Input: part model. Units: mm. Frame: model coordinates. Face numbers are marked on the shaded views. A direction names the side the tool comes from. Coordinates: 2 decimals unless noted, no trailing zeros. Loops run counter-clockwise (first coordinate to the right, second up) from the corner with the lowest first, then second, coordinate; pieces in that order, holes last. Notation, with made-up numbers: (16.5, 70) - (36.5, 70) arc R8 cw to (36.5, 81) - close; hole circle Ø6 at (37.5, 76.5). An arc over 180 degrees is marked (long way). Use a Markdown table: item, result. Add a question column.
1. Ray query, L1, parallel to Z at x = 41, y = -11 (3 decimals); L2, parallel to Z at x = -18, y = -16 (3 decimals); L3, parallel to X at y = -9, z = 42 (3 decimals). Return the intervals inside material, ascending. Write a range as [from, to].
2. Section query B-B on x = 0. Return the cut outline in (y, z) (1 decimal).
3. Section query C-C on z = 33.5. Return the cut outline in (x, y) (3 decimals), then the cut area to 3 significant figures.
4. Access query for the marked faces 1 and 2. Directions: +Z, -Z, +X, -X, +Y, -Y. A direction counts if a zero-diameter tool reaches every point of the face in a straight line with its end or side. Return the directions, or none.
5. Contact query for flat-ended pins moving along their axis: P1, Ø0.8, axis at x = 37, z = -71.5, coming from the -Y side; P2, Ø3, axis at x = 35, z = 72, coming from the -Y side; P3, Ø11, axis at y = -12.5, z = 66, coming from the -X side. Output: stop coordinate, or through.
6. Section query A-A on y = -7. Return the cut outline in (x, z) (3 decimals).
7. Draft query along X for the marked faces 3, 4 and 5. Return one class per face: released by +X, released by -X, zero draft, split by the parting line, or undercut.
```python
from build123d import *

# Parameters (mm, degrees)
SKETCH1_W               = 107.95
SKETCH1_H               = 146.05
BOSS_EXTRUDE1_DEPTH     = 2.54
SKETCH13_W              = 25.4
SKETCH13_H              = 25.4
BOSS_EXTRUDE4_DEPTH     = 19.431
SKETCH2_R               = 3.302
CUT_EXTRUDE1_DEPTH      = 93.862882849
FILLET1_R               = 12.7
CUT_EXTRUDE13_DEPTH     = 5.08
SKETCH15_R              = 6.35
BOSS_EXTRUDE5_DEPTH     = 11.811
SKETCH23_R              = 2.25
CUT_EXTRUDE14_DEPTH     = 92.934228941
SKETCH24_R              = 4
CUT_EXTRUDE15_DEPTH     = 3.81
MIRROR2_COPY_1_SKETCH_R = 2.25
MIRROR2_COPY_1_DEPTH    = 92.934228941
MIRROR2_COPY_2_SKETCH_R = 4
MIRROR2_COPY_2_DEPTH    = 3.81
FILLET3_R               = 12.7
FILLET4_R               = 1.016
SKETCH27_W              = 71.841582164
SKETCH27_H              = 2.54
SKETCH27_W_2            = 2.54
SKETCH27_H_2            = 108.293882364
BOSS_EXTRUDE6_DEPTH     = 33.782
CUT_EXTRUDE16_DEPTH     = 41.656
CUT_EXTRUDE17_DEPTH     = 136.296492227
CUT_EXTRUDE18_DEPTH     = 160.8849299
CUT_EXTRUDE19_REACH     = 161.885
SKETCH31_W              = 22.225
SKETCH31_H              = 12.7
FILLET5_R               = 2.54


with BuildPart() as part:
    # Sketch1 → Boss-Extrude1 (new body)
    with BuildSketch(Plane(origin=(0, 0, 0), x_dir=(1, 0, 0), z_dir=(0, 1, 0))):
        Rectangle(SKETCH1_W, SKETCH1_H)
    extrude(amount=-BOSS_EXTRUDE1_DEPTH)

    # Sketch13 → Boss-Extrude4 (add)
    with BuildSketch(Plane(origin=(0, 0, 0), x_dir=(1, 0, 0), z_dir=(0, 1, 0))):
        with Locations((41.275, -60.325)):
            Rectangle(SKETCH13_W, SKETCH13_H)
        with Locations((-41.275, -60.325)):
            Rectangle(SKETCH13_W, SKETCH13_H)
        with Locations((-41.275, 60.325)):
            Rectangle(SKETCH13_W, SKETCH13_H)
        with Locations((41.275, 60.325)):
            Rectangle(SKETCH13_W, SKETCH13_H)
    extrude(amount=-BOSS_EXTRUDE4_DEPTH)

    # Sketch2 → Cut-Extrude1 (cut, through all)
    with BuildSketch(Plane(origin=(0, 0, 0), x_dir=(1, 0, 0), z_dir=(0, 1, 0))):
        with Locations(Location((-41.275, 60.325, 0), (0, 0, 270))):
            Circle(SKETCH2_R)
        with Locations(Location((41.275, 60.325, 0), (0, 0, 90))):
            Circle(SKETCH2_R)
        with Locations(Location((41.275, -60.325, 0), (0, 0, 270))):
            Circle(SKETCH2_R)
        with Locations(Location((-41.275, -60.325, 0), (0, 0, 90))):
            Circle(SKETCH2_R)
    extrude(amount=-CUT_EXTRUDE1_DEPTH, mode=Mode.SUBTRACT)

    # Fillet1
    fillet1_edges = [part.edges().sort_by_distance(p)[0] for p in [
        (53.975, -9.7155, 73.025),
        (-53.975, -9.7155, 73.025),
        (-53.975, -9.7155, -73.025),
        (53.975, -9.7155, -73.025),
    ]]
    fillet(fillet1_edges, radius=FILLET1_R)

    # Sketch14 → Cut-Extrude13 (cut)
    with BuildSketch(Plane.XZ.offset(19.431)):
        Polygon((20.692003582, -28.674172721), (6.35, -45.983487389), (139.336989519, -156.172707277), (153.678993101, -138.863392609), align=None)
        Polygon((-20.692003582, -28.674172721), (-6.35, -45.983487389), (-139.336989519, -156.172707277), (-153.678993101, -138.863392609), align=None)
        Polygon((-153.678993101, 138.863392609), (-20.692003582, 28.674172721), (-6.35, 45.983487389), (-139.336989519, 156.172707277), align=None)
        Polygon((20.692003582, 28.674172721), (6.35, 45.983487389), (139.336989519, 156.172707277), (153.678993101, 138.863392609), align=None)
    extrude(amount=-CUT_EXTRUDE13_DEPTH, mode=Mode.SUBTRACT)

    # Sketch15 → Boss-Extrude5 (add)
    with BuildSketch(Plane(origin=(0, 0, 0), x_dir=(1, 0, 0), z_dir=(0, 1, 0))):
        with Locations((-41.275, 60.325)):
            Circle(SKETCH15_R)
        with Locations((41.275, 60.325)):
            Circle(SKETCH15_R)
        with Locations((-41.275, -60.325)):
            Circle(SKETCH15_R)
        with Locations((41.275, -60.325)):
            Circle(SKETCH15_R)
    extrude(amount=-BOSS_EXTRUDE5_DEPTH)

    # Sketch23 → Cut-Extrude14 (cut, through all)
    with BuildSketch(Plane.XZ.offset(14.351)):
        with Locations(Location((-41.275, -60.325, 0), (0, 0, 270))):
            Circle(SKETCH23_R)
    cut_extrude14 = extrude(amount=-CUT_EXTRUDE14_DEPTH, mode=Mode.SUBTRACT)

    # Sketch24 → Cut-Extrude15 (cut)
    with BuildSketch(Plane(origin=(0, 0, 0), x_dir=(1, 0, 0), z_dir=(0, 1, 0))):
        with Locations(Location((-41.275, 60.325, 0), (0, 0, 270))):
            Circle(SKETCH24_R)
    cut_extrude15 = extrude(amount=-CUT_EXTRUDE15_DEPTH, mode=Mode.SUBTRACT)

    # Mirror1: Cut-Extrude14, Cut-Extrude15 across plane
    add(cut_extrude14.mirror(Plane.XY), mode=Mode.SUBTRACT)
    add(cut_extrude15.mirror(Plane.XY), mode=Mode.SUBTRACT)

    # Mirror2: Cut-Extrude14, Cut-Extrude15 across plane
    add(cut_extrude14.mirror(Plane(origin=(0, 0, 0), x_dir=(0, 0, 1), z_dir=(1, 0, 0))), mode=Mode.SUBTRACT)
    add(cut_extrude15.mirror(Plane(origin=(0, 0, 0), x_dir=(0, 0, 1), z_dir=(1, 0, 0))), mode=Mode.SUBTRACT)

    # Mirror2 copy 1 sketch → Mirror2 copy 1 (cut, through all)
    with BuildSketch(Plane(origin=(0, -14.351, 0), x_dir=(-1, 0, 0), z_dir=(0, -1, 0))):
        with Locations(Location((-41.275, -60.325, 0), (0, 0, 270))):
            Circle(MIRROR2_COPY_1_SKETCH_R)
    extrude(amount=-MIRROR2_COPY_1_DEPTH, mode=Mode.SUBTRACT)

    # Mirror2 copy 2 sketch → Mirror2 copy 2 (cut)
    with BuildSketch(Plane(origin=(0, 0, 0), x_dir=(-1, 0, 0), z_dir=(0, 1, 0))):
        with Locations(Location((-41.275, 60.325, 0), (0, 0, 270))):
            Circle(MIRROR2_COPY_2_SKETCH_R)
    extrude(amount=-MIRROR2_COPY_2_DEPTH, mode=Mode.SUBTRACT)

    # Fillet3
    fillet3_edges = [part.edges().sort_by_distance(p)[0] for p in [
        (28.575, -8.4455, -47.625),
        (-28.575, -8.4455, -47.625),
        (-28.575, -8.4455, 47.625),
        (28.575, -8.4455, 47.625),
    ]]
    fillet(fillet3_edges, radius=FILLET3_R)

    # Fillet4
    fillet4_edges = [part.edges().sort_by_distance(p)[0] for p in [
        (41.275, -14.351, -57.023),
        (-41.275, -14.351, -63.627),
        (-41.275, -14.351, 63.627),
        (41.275, -14.351, 57.023),
    ]]
    fillet(fillet4_edges, radius=FILLET4_R)

    # Sketch27 → Boss-Extrude6 (add)
    with BuildSketch(Plane.XZ.offset(2.54)):
        with Locations((0, -71.755)):
            Rectangle(SKETCH27_W, SKETCH27_H)
        with Locations((0, 71.755)):
            Rectangle(SKETCH27_W, SKETCH27_H)
        with Locations((52.705, 0)):
            Rectangle(SKETCH27_W_2, SKETCH27_H_2)
        with Locations((-52.705, 0)):
            Rectangle(SKETCH27_W_2, SKETCH27_H_2)
    extrude(amount=BOSS_EXTRUDE6_DEPTH)

    # Sketch28 → Cut-Extrude16 (cut)
    with BuildSketch(Plane(origin=(0, 0, -73.025), x_dir=(-1, 0, 0), z_dir=(0, 0, -1))):
        with BuildLine():
            Line((-17.526, -36.322), (17.526, -36.322))
            Line((17.526, -36.322), (29.591, -36.322))
            Line((29.591, -36.322), (29.591, -33.782))
            ThreePointArc((29.591, -33.782), (28.847051224, -31.985948776), (27.051, -31.242))
            Line((27.051, -31.242), (19.431, -31.242))
            ThreePointArc((19.431, -31.242), (17.634948776, -30.498051224), (16.891, -28.702))
            Line((16.891, -28.702), (16.891, -21.3995))
            ThreePointArc((16.891, -21.3995), (16.147051224, -19.603448776), (14.351, -18.8595))
            Line((14.351, -18.8595), (-14.351, -18.8595))
            ThreePointArc((-14.351, -18.8595), (-16.147051224, -19.603448776), (-16.891, -21.3995))
            Line((-16.891, -21.3995), (-16.891, -28.702))
            ThreePointArc((-16.891, -28.702), (-17.634948776, -30.498051224), (-19.431, -31.242))
            Line((-19.431, -31.242), (-27.051, -31.242))
            ThreePointArc((-27.051, -31.242), (-28.847051224, -31.985948776), (-29.591, -33.782))
            Line((-29.591, -33.782), (-29.591, -36.322))
            Line((-29.591, -36.322), (-17.526, -36.322))
        make_face()
    extrude(amount=-CUT_EXTRUDE16_DEPTH, mode=Mode.SUBTRACT)

    # Sketch29 → Cut-Extrude17 (cut, through all)
    with BuildSketch(Plane.ZY.offset(53.975)):
        with BuildLine():
            Line((-54.146941182, -36.322), (-49.066941182, -36.322))
            Line((-49.066941182, -36.322), (-49.066941182, -33.782))
            ThreePointArc((-49.066941182, -33.782), (-49.810889958, -31.985948776), (-51.606941182, -31.242))
            Line((-51.606941182, -31.242), (-54.146941182, -31.242))
            Line((-54.146941182, -31.242), (-54.146941182, -36.322))
        make_face()
        with BuildLine():
            Line((49.066941182, -36.322), (49.066941182, -33.782))
            ThreePointArc((49.066941182, -33.782), (49.810889958, -31.985948776), (51.606941182, -31.242))
            Line((51.606941182, -31.242), (54.146941182, -31.242))
            Line((54.146941182, -31.242), (54.146941182, -36.322))
            Line((54.146941182, -36.322), (49.066941182, -36.322))
        make_face()
    extrude(amount=-CUT_EXTRUDE17_DEPTH, mode=Mode.SUBTRACT)

    # Sketch30 → Cut-Extrude18 (cut, through all)
    with BuildSketch(Plane.XY.offset(73.025)):
        with BuildLine():
            Line((-35.920791082, -36.322), (-30.840791082, -36.322))
            Line((-30.840791082, -36.322), (-30.840791082, -33.782))
            ThreePointArc((-30.840791082, -33.782), (-31.584739858, -31.985948776), (-33.380791082, -31.242))
            Line((-33.380791082, -31.242), (-35.920791082, -31.242))
            Line((-35.920791082, -31.242), (-35.920791082, -36.322))
        make_face()
        with BuildLine():
            Line((30.840791082, -36.322), (30.840791082, -33.782))
            ThreePointArc((30.840791082, -33.782), (31.584739858, -31.985948776), (33.380791082, -31.242))
            Line((33.380791082, -31.242), (35.920791082, -31.242))
            Line((35.920791082, -31.242), (35.920791082, -36.322))
            Line((35.920791082, -36.322), (30.840791082, -36.322))
        make_face()
    extrude(amount=-CUT_EXTRUDE18_DEPTH, mode=Mode.SUBTRACT)

    # Sketch31 → Cut-Extrude19 (cut, up to next)
    with BuildSketch(Plane.XY.offset(73.025), mode=Mode.PRIVATE) as cut_extrude19_sk1:
        with Locations((0, -29.972)):
            Rectangle(SKETCH31_W, SKETCH31_H)
    cut_extrude19_tool1 = extrude(cut_extrude19_sk1.sketch, amount=-CUT_EXTRUDE19_REACH, mode=Mode.PRIVATE) & part.part
    add(cut_extrude19_tool1.solids().sort_by_distance((0, -29.972, 73.025))[0], mode=Mode.SUBTRACT)

    # Fillet5
    fillet5_edges = [part.edges().sort_by_distance(p)[0] for p in [
        (-11.1125, -23.622, 71.755),
        (11.1125, -23.622, 71.755),
    ]]
    fillet(fillet5_edges, radius=FILLET5_R)


solid = part.part
```
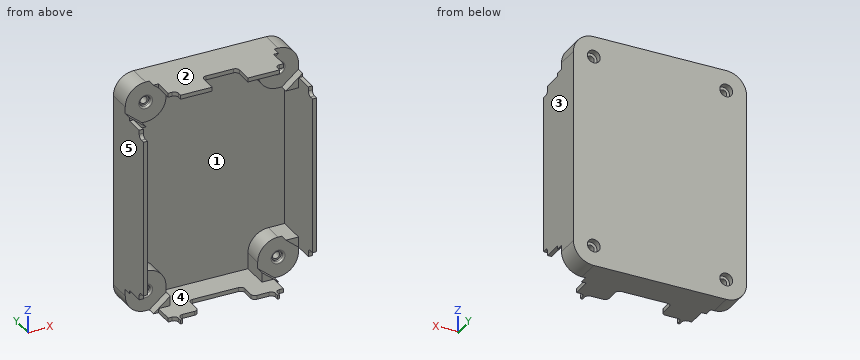
Resolved:
| question | item | result |
|---|---|---|
| 1 | L1 | [-73.025, -62.558], [-58.092, -47.628], [47.628, 58.092], [62.558, 73.025] |
| 1 | L2 | [-73.025, -70.485], [70.485, 73.025] |
| 1 | L3 | [-53.975, -51.435], [51.435, 53.975] |
| 2 | outline | (-23.6, 70.5) - (-2.5, 70.5) - (-2.5, -70.5) - (-18.9, -70.5) - (-18.9, -73) - (0, -73) - (0, 73) - (-23.6, 73) - close |
| 3 | outline | (-53.975, -36.322) - (-51.435, -36.322) - (-51.435, -2.54) - (51.435, -2.54) - (51.435, -36.322) - (53.975, -36.322) - (53.975, 0) - (-53.975, 0) - close |
| 3 | area | 446 mm² |
| 4 | face 1 | -Y |
| 4 | face 2 | +Z, +X, -X, +Y, -Y |
| 5 | P1 | y = -19.43 |
| 5 | P2 | y = -31.24 |
| 5 | P3 | x = -53.97 |
| 6 | outline | (-53.975, -60.325) arc R12.7 ccw to (-41.275, -73.025) - (41.275, -73.025) arc R12.7 ccw to (53.975, -60.325) - (53.975, 60.325) arc R12.7 ccw to (41.275, 73.025) - (-41.275, 73.025) arc R12.7 ccw to (-53.975, 60.325) - close; hole (-51.435, -47.625) - (-41.275, -47.625) arc R12.7 cw to (-28.575, -60.325) - (-28.575, -70.485) - (28.575, -70.485) - (28.575, -60.325) arc R12.7 cw to (41.275, -47.625) - (51.435, -47.625) - (51.435, 47.625) - (41.275, 47.625) arc R12.7 cw to (28.575, 60.325) - (28.575, 70.485) - (-28.575, 70.485) - (-28.575, 60.325) arc R12.7 cw to (-41.275, 47.625) - (-51.435, 47.625) - close; hole circle Ø4.5 at (-41.275, -60.325); hole circle Ø4.5 at (-41.275, 60.325); hole circle Ø4.5 at (41.275, -60.325); hole circle Ø4.5 at (41.275, 60.325) |
| 7 | face 3 | released by +X |
| 7 | face 4 | undercut |
| 7 | face 5 | released by -X |
